Drawing for the job (mm, zero at the part's lowest x, y, z). A direction names the side the tool comes from. Coordinates: 2 decimals unless noted, no trailing zeros. Loops run counter-clockwise (first coordinate to the right, second up) from the corner with the lowest first, then second, coordinate; pieces in that order, holes last. Notation, with made-up numbers: (2, 5) - (15, 5) arc R5 cw to (15, 10) - close; hole circle Ø6 at (22.25, 57.5). An arc over 180 degrees is marked (long way). One line per item, written item: value.
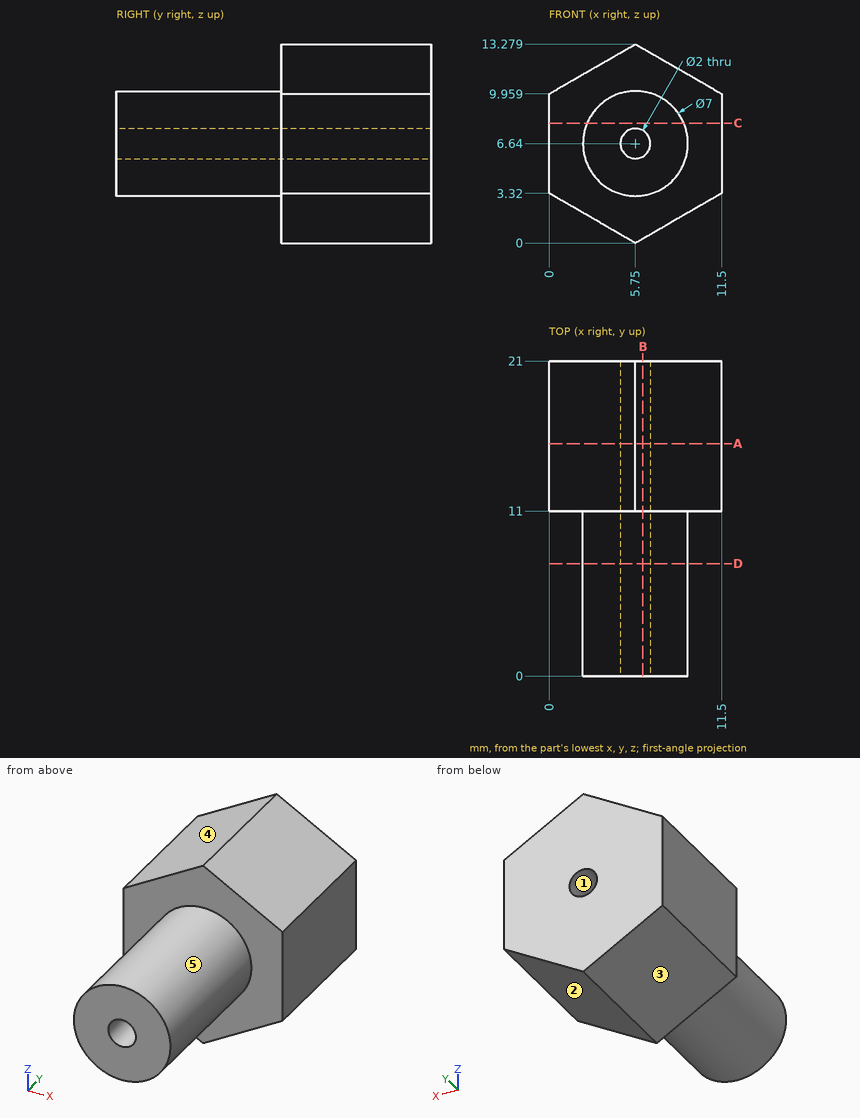
Item 1: Cut at A-A, the plane y = 15.5. Write the cut outline in (x, z).
Check result:
outline: (0, 3.32) - (5.75, 0) - (11.5, 3.32) - (11.5, 9.96) - (5.75, 13.28) - (0, 9.96) - close; hole circle Ø2 at (5.75, 6.64)
Item 2: Cut at C-C, the plane z = 8. Write the cut outline in (x, y) (1 decimal), then the cut area to 3 significant figures.
Check result:
outline: (0, 11) - (2.5, 11) - (2.5, 0) - (9, 0) - (9, 11) - (11.5, 11) - (11.5, 21) - (0, 21) - close
area: 186 mm^2
Item 3: Pull direction X, two halves, no side cores. Call the marked faces 1, 2 and 3: released by +X, released by -X, zero draft, split by the parting line, or undercut.
Check result:
face 1: undercut
face 2: released by +X
face 3: released by -X
Item 4: Cut at D-D, the plane y = 7.5. Write the cut outline in (x, z).
Check result:
outline: circle Ø7 at (5.75, 6.64); hole circle Ø2 at (5.75, 6.64)
Item 5: Cut at B-B, the plane x = 6.25. Write the cut outline in (y, z) (1 decimal), then the cut area to 3 significant figures.
Check result:
outline: (0, 3.2) - (11, 3.2) - (11, 0.3) - (21, 0.3) - (21, 5.8) - (0, 5.8) - close; (0, 7.5) - (21, 7.5) - (21, 13) - (11, 13) - (11, 10.1) - (0, 10.1) - close
area: 167 mm^2
Item 6: Tool access for the marked faces 4 and 5: list every direction of +Z, -Z, +X, -X, +Y, -Y with a clear straight run to the whole face (end or side of a thin tool).
Check result:
face 4: +Z, -X, +Y, -Y
face 5: -Y
Item 7: Probe probe 1 along Y at (x, z) = (9.75, 5.5); probe 2 along X at (y, z) = (12.5, 7.25); probe 3 along Z at (x, y) = (5, 3) (1 decimal). List the from-to ranges inside material, lowest first. Write a range as from..to.
Check result:
probe 1: y = 11..21
probe 2: x = 0..4.96, 6.54..11.5
probe 3: z = 3.2..6, 7.3..10.1
Item 8: Drop flat-ended pins along their axis: P1, Ø2, axis at x = 9, z = 10.5, coming from the -Y side; P2, Ø5, axis at x = 9, y = 4, coming from the -Z side; P3, Ø3, axis at y = 16.5, z = 1.5, coming from the -X side (1 decimal). Give the stop position or say it passes through.
Check result:
P1: stops at y = 11
P2: stops at z = 3.22
P3: stops at x = 0.6
